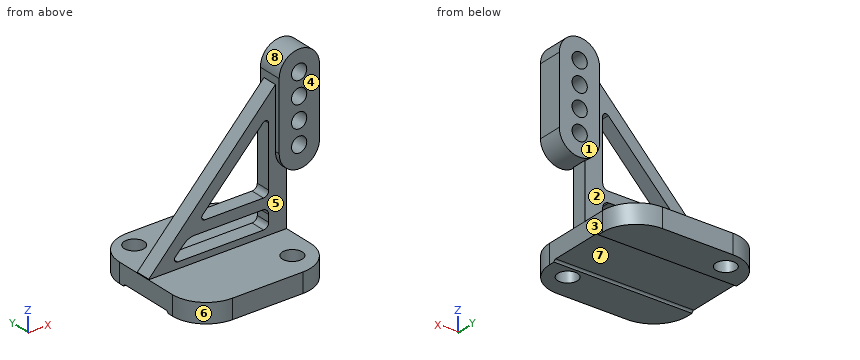
from build123d import *

# Parameters (mm, degrees)
PAD_DEPTH       = 8
POCKET_DEPTH    = 57.0073705793
SKETCH002_R     = 4.0836886852
POCKET001_DEPTH = 8.001
SKETCH003_W     = 56.899337
SKETCH003_H     = 6.084113
PAD001_DEPTH    = 60
POCKET002_DEPTH = 29.4027415793
POCKET003_DEPTH = 29.4027415793
PAD002_DEPTH    = 5
SKETCH007_R     = 3.14062
POCKET004_DEPTH = 31.4027415793


with BuildPart() as part:
    # Sketch → Pad (new body)
    with BuildSketch(Plane.XY):
        with BuildLine():
            ThreePointArc((-15.0477684207, 26.4331275793), (-24.9562751358, 22.3288897151), (-29.060513, 12.420383))
            Line((-29.060513, -15.6050894207), (-29.060513, 12.420383))
            ThreePointArc((-29.060513, -15.6050894207), (-24.9562751358, -25.5135961358), (-15.0477684207, -29.617834))
            Line((13.933113, -29.617834), (-15.0477684207, -29.617834))
            ThreePointArc((13.933113, -29.617834), (23.841619715, -25.5135961358), (27.9458575793, -15.6050894207))
            Line((27.9458575793, 12.420383), (27.9458575793, -15.6050894207))
            ThreePointArc((27.9458575793, 12.420383), (23.8416197151, 22.3288897151), (13.933113, 26.4331275793))
            Line((-15.0477684207, 26.4331275793), (13.933113, 26.4331275793))
        make_face()
    extrude(amount=PAD_DEPTH)

    # Sketch001 (on Face6 of Pad) → Pocket (cut, through all)
    with BuildSketch(Plane.YZ.offset(27.9458575793)):
        with BuildLine():
            ThreePointArc((-12.380569, 0.7961803172), (-13.0279997287, 0.5280057287), (-13.2961743172, -0.119425))
            Line((-13.2961743172, -1.9506356828), (-13.2961743172, -0.119425))
            ThreePointArc((-13.2961743172, -1.9506356828), (-13.0279997287, -2.5980664115), (-12.380569, -2.866241))
            Line((9.355097, -2.866241), (-12.380569, -2.866241))
            ThreePointArc((9.355097, -2.866241), (10.0025277287, -2.5980664115), (10.2707023172, -1.9506356828))
            Line((10.2707023172, -0.119425), (10.2707023172, -1.9506356828))
            ThreePointArc((10.2707023172, -0.119425), (10.0025277287, 0.5280057287), (9.355097, 0.7961803172))
            Line((-12.380569, 0.7961803172), (9.355097, 0.7961803172))
        make_face()
    extrude(amount=-POCKET_DEPTH, mode=Mode.SUBTRACT)

    # Sketch002 (on Face5 of Pocket) → Pocket001 (cut, through all)
    with BuildSketch(Plane.XY.offset(8)):
        with Locations((-18.148907, 18.645535)):
            Circle(SKETCH002_R)
        with Locations((18.148907, -18.645535)):
            Circle(SKETCH002_R)
    extrude(amount=-POCKET001_DEPTH, mode=Mode.SUBTRACT)

    # Sketch003 (on Face5 of Pocket001) → Pad001 (join)
    with BuildSketch(Plane.XY.offset(8)):
        with Locations((-0.5137005, 0.0734425)):
            Rectangle(SKETCH003_W, SKETCH003_H)
    extrude(amount=PAD001_DEPTH)

    # Sketch004 (on Face18 of Pad001) → Pocket002 (cut, through all)
    with BuildSketch(Plane.XZ.offset(2.968614)):
        Polygon((32.25227, 72.310852), (-33.045937, 3.912876), (-33.045937, 72.310852), align=None)
    extrude(amount=-POCKET002_DEPTH, mode=Mode.SUBTRACT)

    # Sketch005 (on Face18 of Pocket002) → Pocket003 (cut, through all)
    with BuildSketch(Plane.XZ.offset(2.968614)):
        with BuildLine():
            Line((20.576633, 49.5814919899), (20.576633, 24.688993))
            ThreePointArc((18.39756, 22.50992), (19.938397295, 23.148155705), (20.576633, 24.688993))
            Line((18.39756, 22.50992), (-5.8443663857, 22.50992))
            ThreePointArc((-6.7417037948, 24.6225852162), (-6.992034537, 23.2693582646), (-5.8443663857, 22.50992))
            Line((-6.7417037948, 24.6225852162), (18.2466667899, 50.5222462275))
            ThreePointArc((20.576633, 49.5814919899), (19.7290007026, 50.837851918), (18.2466667899, 50.5222462275))
        make_face()
        with BuildLine():
            Line((-14.3464422841, 16.4193365685), (-17.9321506281, 12.8610900081))
            ThreePointArc((-17.9321506281, 12.8610900081), (-18.2216862616, 11.4271148765), (-17.0060998632, 10.6131951821))
            Line((-17.0060998632, 10.6131951821), (18.45566, 10.6131951821))
            ThreePointArc((18.45566, 10.6131951821), (19.955414391, 11.234413791), (20.576633, 12.7341681821))
            Line((20.576633, 12.7341681821), (20.576633, 15.643153))
            ThreePointArc((20.576633, 15.643153), (19.8342365583, 17.4354565583), (18.041933, 18.177853))
            Line((18.041933, 18.177853), (-10.0778210188, 18.177853))
            ThreePointArc((-10.0778210188, 18.177853), (-12.3861487439, 17.7210037241), (-14.3464422841, 16.4193365685))
        make_face()
    extrude(amount=-POCKET003_DEPTH, mode=Mode.SUBTRACT)

    # Sketch006 (on Face18 of Pocket003) → Pad002 (join, symmetric)
    with BuildSketch(Plane.XZ.offset(-0.031386)):
        with BuildLine():
            ThreePointArc((39.9948353179, 65.999481), (31.665817, 74.3284993179), (23.3367986821, 65.999481))
            Line((23.3367986821, 65.999481), (23.3367986821, 38.133236))
            ThreePointArc((23.3367986821, 38.133236), (31.665817, 29.8042176821), (39.9948353179, 38.133236))
            Line((39.9948353179, 38.133236), (39.9948353179, 65.999481))
        make_face()
    extrude(amount=PAD002_DEPTH, both=True)

    # Sketch007 (on Face39 of Pad002) → Pocket004 (cut, through all)
    with BuildSketch(Plane.XZ.offset(4.968614)):
        with Locations((31.585516, 65.792679)):
            Circle(SKETCH007_R)
        with Locations((31.585516, 56.792679)):
            Circle(SKETCH007_R)
        with Locations((31.585516, 47.792679)):
            Circle(SKETCH007_R)
        with Locations((31.585516, 38.792679)):
            Circle(SKETCH007_R)
    extrude(amount=-POCKET004_DEPTH, mode=Mode.SUBTRACT)


solid = part.part
Build history of the part. All positions in model axes, mm. Face numbers are marked on the shaded views. A direction names the side the tool comes from. Round coordinates to 2 decimals unless told otherwise and drop trailing zeros. Write each loop counter-clockwise with the first axis right and the second up, starting at its lowest first coordinate (ties: lowest second). Pieces come first, ordered by that corner, then holes. Notation, with made-up numbers: (89, 55) -> (133, 55) arc R23 ccw to (133, 90) -> close; hole circle Ø8 at (-15.75, -13.5). An arc over 180 degrees is marked (long way). Write item = value, one per line.
(1) Band-saw the part on A-A (z = 67). Give the cut face in (x, y), then the cut area to 3 significant figures.
Answer:
outline = (23.4, -4.97) -> (28.69, -4.97) -> (28.69, 5.03) -> (23.4, 5.03) -> close; (34.48, -4.97) -> (39.93, -4.97) -> (39.93, 5.03) -> (34.48, 5.03) -> close
area = 107 mm2
(2) Band-saw the part on D-D (x = 30.5). Give the cut face in (y, z), then the cut area to 3 significant figures.
Answer:
outline = (-4.97, 29.89) -> (5.03, 29.89) -> (5.03, 35.85) -> (-4.97, 35.85) -> close; (-4.97, 41.74) -> (5.03, 41.74) -> (5.03, 44.85) -> (-4.97, 44.85) -> close; (-4.97, 50.74) -> (5.03, 50.74) -> (5.03, 53.85) -> (-4.97, 53.85) -> close; (-4.97, 59.74) -> (5.03, 59.74) -> (5.03, 62.85) -> (-4.97, 62.85) -> close; (-4.97, 68.74) -> (5.03, 68.74) -> (5.03, 74.25) -> (-4.97, 74.25) -> close
area = 208 mm2
(3) Tool access for the marked faces 1, 2, 3 and 4: list every direction of +Z, -Z, +X, -X, +Y, -Y with a clear straight run to the whole face (end or side of a thin tool).
Answer:
face_1 = +Z, +X, -X, +Y
face_2 = -X, +Y
face_3 = -Z, +X, +Y, -Y
face_4 = +Z, +X, -X, -Y
(4) Band-saw the part on B-B (x = 4.5). Give the cut face in (y, z), then the cut area to 3 significant figures.
Answer:
outline = (-29.62, 0) -> (-13.29, 0) arc R0.92 cw to (-12.38, 0.8) -> (9.36, 0.8) arc R0.92 cw to (10.26, 0) -> (26.43, 0) -> (26.43, 8) -> (3.12, 8) -> (3.12, 10.61) -> (-2.97, 10.61) -> (-2.97, 8) -> (-29.62, 8) -> close; (-2.97, 18.18) -> (3.12, 18.18) -> (3.12, 22.51) -> (-2.97, 22.51) -> close; (-2.97, 36.27) -> (3.12, 36.27) -> (3.12, 43.24) -> (-2.97, 43.24) -> close
area = 515 mm2
(5) Probe L1, parallel to X at y = 1.5, z = 37; L2, parallel to Z at x = -3, y = 1; L3, parallel to Z at x = 17.5, y = 2. List the from-to ranges inside material, lowest first.
Answer:
L1 = -1.46 to 5.2, 20.58 to 29.01, 34.16 to 39.92
L2 = 0.8 to 10.61, 18.18 to 22.51, 28.5 to 35.39
L3 = 0.8 to 10.61, 18.18 to 22.51, 49.75 to 56.86
(6) Two-plate mould, pull along Z, no slides. Class the marked faces 5, 6, 7 and 8: pulls with the +Z half, pulls with the -Z half, needs draft (parallel to the pull), parting line crosses it, or undercut.
Answer:
face_5 = undercut
face_6 = needs draft
face_7 = pulls with the -Z half
face_8 = pulls with the +Z half
(7) Band-saw the part on C-C (y = 21.5). Give the cut face in (x, z), then the cut area to 3 significant figures.
Answer:
outline = (-25.72, 0) -> (-21.07, 0) -> (-21.07, 8) -> (-25.72, 8) -> close; (-15.23, 0) -> (24.61, 0) -> (24.61, 8) -> (-15.23, 8) -> close
area = 356 mm2
(8) Flat gauge pins, fed straight in: pin 1 (8 mm diameter, centred on y = -7, z = 30.5, fed in from +X); pin 2 (6 mm diameter, centred on x = 22, z = 33, fed in from -Y); pin 3 (10 mm diameter, centred on x = 31.59, z = 65.79, fed in from +Y). Where does each tip first touch, or does it go through?
Answer:
pin_1 = 38.87
pin_2 = -4.97
pin_3 = 5.03
